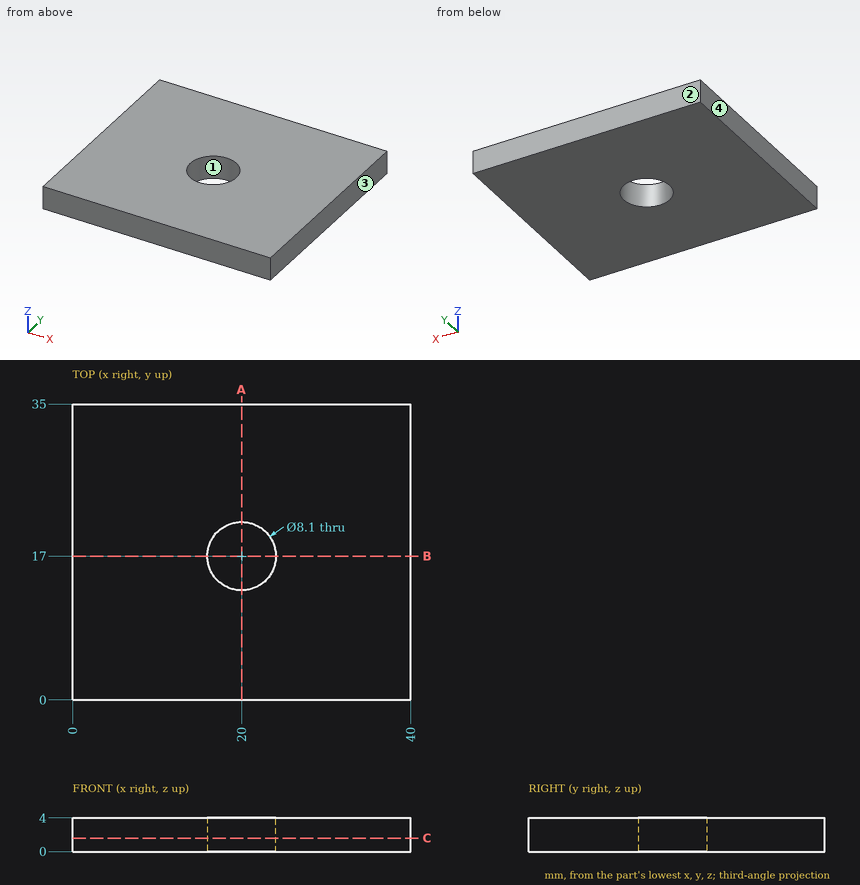
The drawing under review shows one solid part. Ordinate dimensions are in mm from its lowest x, y, z. Round coordinates to 2 decimals unless told otherwise and drop trailing zeros. Loops run counter-clockwise (first coordinate to the right, second up) from the corner with the lowest first, then second, coordinate; pieces in that order, holes last. Notation, with made-up numbers: M 70,-22.75 L 84,-22.75 A13 cw 84,-8.75 Z; hole C 24,4 d9. An arc over 180 degrees is marked long. Answer as CSV lines item,"result". Start each with the question number.
Item 1: Wall thickness on line 1 (X direction, y = 17, z = 3.25); line 2 (Y direction, x = 20, z = 2.75); line 3 (X direction, y = 14.5, z = 2.1): over which ranges is each line inside the solid? List them lowest first. Write a range as [from, to].
Item 2: Insertion check: P1, Ø13, axis at x = 20, y = 17, coming from the +Z side. The pin has a flat end and moves straight along its axis. Give the tip position at first contact, or say it passes through.
Item 3: Mouldability with a two-part tool opening along X and no side actions: class the marked faces 1, 2, 3 and 4 as released by +X, released by -X, zero draft, split by the parting line, or undercut.
Item 4: Consider section A-A (x = 20). Write out the cut boundary in (y, z).
Item 5: Consider section C-C (z = 1.6). Write out the cut boundary in (x, y), then the cut area to 3 significant figures.
Item 6: Consider section B-B (y = 17). Write out the cut boundary in (x, z).
Answer:
1,line 1,"x = [0, 15.95], [24.05, 40]"
1,line 2,"y = [0, 12.95], [21.05, 35]"
1,line 3,"x = [0, 16.81], [23.19, 40]"
2,P1,"stops at z = 4"
3,face 1,"undercut"
3,face 2,"zero draft"
3,face 3,"released by +X"
3,face 4,"released by -X"
4,outline,"M 0,0 L 12.95,0 L 12.95,4 L 0,4 Z; M 21.05,0 L 35,0 L 35,4 L 21.05,4 Z"
5,outline,"M 0,0 L 40,0 L 40,35 L 0,35 Z; hole C 20,17 d8.1"
5,area,"1,350 mm^2"
6,outline,"M 0,0 L 15.95,0 L 15.95,4 L 0,4 Z; M 24.05,0 L 40,0 L 40,4 L 24.05,4 Z"
